Work out the finished part from the listing and answer in its coordinate system (mm). A direction names the side the tool comes from. Give positions to 0.01 mm unless a question says otherwise; leave off trailing zeros. Order: outer loops, then holes, each group sorted by start corner. A loop starts at its lowest first (then second) coordinate and runs counter-clockwise, first axis right, second up.
```python
from build123d import *

# Parameters (mm, degrees)
BOSS_EXTRUDE1_DEPTH = 1.2
FILLET1_R           = 4
FILLET2_R           = 2.5
BOSS_EXTRUDE2_DEPTH = 0.9
CUT_EXTRUDE1_DEPTH  = 0.9
CUT_EXTRUDE2_DEPTH  = 86.698804049


with BuildPart() as part:
    # Sketch1 → Boss-Extrude1 (new body)
    with BuildSketch(Plane(origin=(0, 0, 0), x_dir=(1, 0, 0), z_dir=(0, 1, 0))):
        Polygon((-59.653240417, 31.238807945), (-9.653240417, 31.238807945), (-9.653240417, 36.238807945), (-4.653240417, 36.238807945), (-4.653240417, 51.238807945), (-9.653240417, 51.238807945), (-9.653240417, 56.238807945), (-59.653240417, 56.238807945), (-59.653240417, 51.238807945), (-64.653240417, 51.238807945), (-64.653240417, 36.238807945), (-59.653240417, 36.238807945), align=None)
    extrude(amount=BOSS_EXTRUDE1_DEPTH)

    # Fillet1
    fillet1_edges = [part.edges().sort_by_distance(p)[0] for p in [
        (-59.653240417, 0.6, -56.238807945),
        (-9.653240417, 0.6, -56.238807945),
        (-9.653240417, 0.6, -31.238807945),
        (-59.653240417, 0.6, -31.238807945),
    ]]
    fillet(fillet1_edges, radius=FILLET1_R)

    # Fillet2
    fillet2_edges = [part.edges().sort_by_distance(p)[0] for p in [
        (-64.653240417, 0.6, -36.238807945),
        (-64.653240417, 0.6, -51.238807945),
        (-4.653240417, 0.6, -51.238807945),
        (-4.653240417, 0.6, -36.238807945),
    ]]
    fillet(fillet2_edges, radius=FILLET2_R)

    # Sketch4 → Boss-Extrude2 (add)
    with BuildSketch(Plane(origin=(0, 1.2, 0), x_dir=(1, 0, 0), z_dir=(0, 1, 0))):
        with BuildLine():
            Line((-59.153240417, 50.738807945), (-59.153240417, 36.738807945))
            Line((-59.153240417, 36.738807945), (-59.153240417, 35.238807945))
            ThreePointArc((-59.153240417, 35.238807945), (-58.128114151, 32.763934211), (-55.653240417, 31.738807945))
            Line((-55.653240417, 31.738807945), (-13.653240417, 31.738807945))
            ThreePointArc((-13.653240417, 31.738807945), (-11.178366683, 32.763934211), (-10.153240417, 35.238807945))
            Line((-10.153240417, 35.238807945), (-10.153240417, 36.738807945))
            Line((-10.153240417, 36.738807945), (-10.153240417, 50.738807945))
            Line((-10.153240417, 50.738807945), (-10.153240417, 52.238807945))
            ThreePointArc((-10.153240417, 52.238807945), (-11.178366683, 54.713681679), (-13.653240417, 55.738807945))
            Line((-13.653240417, 55.738807945), (-55.653240417, 55.738807945))
            ThreePointArc((-55.653240417, 55.738807945), (-58.128114151, 54.713681679), (-59.153240417, 52.238807945))
            Line((-59.153240417, 52.238807945), (-59.153240417, 50.738807945))
        make_face()
    extrude(amount=BOSS_EXTRUDE2_DEPTH)

    # Sketch5 → Cut-Extrude1 (cut)
    with BuildSketch(Plane(origin=(0, 2.1, 0), x_dir=(1, 0, 0), z_dir=(0, 1, 0))):
        with BuildLine():
            Line((-58.553240417, 52.238807945), (-58.553240417, 35.238807945))
            ThreePointArc((-58.553240417, 35.238807945), (-57.703850082, 33.18819828), (-55.653240417, 32.338807945))
            Line((-55.653240417, 32.338807945), (-13.653240417, 32.338807945))
            ThreePointArc((-13.653240417, 32.338807945), (-11.602630751, 33.18819828), (-10.753240417, 35.238807945))
            Line((-10.753240417, 35.238807945), (-10.753240417, 52.238807945))
            ThreePointArc((-10.753240417, 52.238807945), (-11.602630751, 54.289417611), (-13.653240417, 55.138807945))
            Line((-13.653240417, 55.138807945), (-55.653240417, 55.138807945))
            ThreePointArc((-55.653240417, 55.138807945), (-57.703850082, 54.289417611), (-58.553240417, 52.238807945))
        make_face()
    extrude(amount=-CUT_EXTRUDE1_DEPTH, mode=Mode.SUBTRACT)

    # Sketch6 → Cut-Extrude2 (cut, through all)
    with BuildSketch(Plane(origin=(0, 1.2, 0), x_dir=(1, 0, 0), z_dir=(0, 1, 0))):
        with BuildLine():
            Line((-63.153240417, 48.738807945), (-63.153240417, 38.738807945))
            ThreePointArc((-63.153240417, 38.738807945), (-62.153240417, 37.738807945), (-61.153240417, 38.738807945))
            Line((-61.153240417, 38.738807945), (-61.153240417, 48.738807945))
            ThreePointArc((-61.153240417, 48.738807945), (-62.153240417, 49.738807945), (-63.153240417, 48.738807945))
        make_face()
        with BuildLine():
            Line((-8.153185775, 48.728354232), (-8.153240417, 38.738807945))
            ThreePointArc((-8.153240417, 38.738807945), (-7.153245887, 37.738807945), (-6.153240417, 38.738807945))
            Line((-6.153240417, 38.738807945), (-6.153240417, 48.738807945))
            ThreePointArc((-6.153240417, 48.738807945), (-7.158467345, 49.738794285), (-8.153185775, 48.728354232))
        make_face()
    extrude(amount=-CUT_EXTRUDE2_DEPTH, mode=Mode.SUBTRACT)


solid = part.part
```
1. The part is cut by section C-C (z = -54.25). Write down the section's boundary in (x, y), then the cut area to 3 significant figures.
Findings below:
outline: (-59.11, 0) - (-10.2, 0) - (-10.2, 1.2) - (-10.79, 1.2) - (-10.79, 2.1) - (-11.56, 2.1) - (-11.56, 1.2) - (-57.74, 1.2) - (-57.74, 2.1) - (-58.52, 2.1) - (-58.52, 1.2) - (-59.11, 1.2) - close
area: 60.1 mm2
2. The part is cut by section A-A (y = 0.4). Write down the section's boundary in (x, z).
Findings below:
outline: (-64.65, -48.74) arc R2.5 ccw to (-62.15, -51.24) - (-59.65, -51.24) - (-59.65, -52.24) arc R4 ccw to (-55.65, -56.24) - (-13.65, -56.24) arc R4 ccw to (-9.65, -52.24) - (-9.65, -51.24) - (-7.15, -51.24) arc R2.5 ccw to (-4.65, -48.74) - (-4.65, -38.74) arc R2.5 ccw to (-7.15, -36.24) - (-9.65, -36.24) - (-9.65, -35.24) arc R4 ccw to (-13.65, -31.24) - (-55.65, -31.24) arc R4 ccw to (-59.65, -35.24) - (-59.65, -36.24) - (-62.15, -36.24) arc R2.5 ccw to (-64.65, -38.74) - close; hole (-63.15, -48.74) arc R1 ccw to (-61.15, -48.74) - (-61.15, -38.74) arc R1 ccw to (-63.15, -38.74) - close; hole (-8.15, -48.73) arc R1 ccw (long way) to (-6.15, -48.74) - (-6.15, -38.74) arc R1 ccw to (-8.15, -38.74) - close
3. The part is cut by section D-D (z = -45.25). Write down the section's boundary in (x, y).
Findings below:
outline: (-64.65, 0) - (-63.15, 0) - (-63.15, 1.2) - (-64.65, 1.2) - close; (-61.15, 0) - (-8.15, 0) - (-8.15, 1.2) - (-10.15, 1.2) - (-10.15, 2.1) - (-10.75, 2.1) - (-10.75, 1.2) - (-58.55, 1.2) - (-58.55, 2.1) - (-59.15, 2.1) - (-59.15, 1.2) - (-61.15, 1.2) - close; (-6.15, 0) - (-4.65, 0) - (-4.65, 1.2) - (-6.15, 1.2) - close
4. The mould has two halves that part along Z. Classify faces 6 (the face through (-10.794, 0.608, -55.036)), 7 (the face through (-62.13, 0.61, -49.74)), 8 (the face through (-8, 1, -36.239)): pulls with the +Z half, pulls with the -Z half, needs draft (parallel to the pull), parting line crosses it, or undercut.
Findings below:
face 6: pulls with the -Z half
face 7: undercut
face 8: pulls with the +Z half
5. The part is cut by section B-B (x = -28). Write down the section's boundary in (y, z), then the cut area to 3 significant figures.
Findings below:
outline: (0, -56.24) - (1.2, -56.24) - (1.2, -55.74) - (2.1, -55.74) - (2.1, -55.14) - (1.2, -55.14) - (1.2, -32.34) - (2.1, -32.34) - (2.1, -31.74) - (1.2, -31.74) - (1.2, -31.24) - (0, -31.24) - close
area: 31.1 mm2
6. Given P1, Ø0.6, axis at x = -61, y = 1, coming from the -Z side; P2, Ø0.5, axis at x = -34.5, y = 1.5, coming from the +Z side; P3, Ø1, axis at x = -26, z = -45, coming from the +Y side, each flat-ended and moving along its own axis, determine where each tip first touches the part or whether it passes through.
Findings below:
P1: stops at z = -51.24
P2: stops at z = -31.74
P3: stops at y = 1.2
7. Which of the six approach directions +Z, -Z, +X, -X, +Y, -Y give full straight-line access (tool end or side, diameter ignored) to faces 1 (the face through (-7.18, 0.61, -37.74)), 2 (the face through (-11.206, 1.644, -32.737)), 3 (the face through (-61, 1, -51.239)), 4 (the face through (-11.151, 1.644, -54.686)), 5 (the face through (-35, 1.2, -44))?
Findings below:
face 1: +Y, -Y
face 2: +Z, +X, +Y
face 3: -Z, -X, +Y, -Y
face 4: -Z, +X, +Y
face 5: +Y
8. Straight lines are drawn through the part: probe 1 along X at (y, z) = (0.1, -40.75); probe 2 along Z at (x, y) = (-28, 1.6); probe 3 along X at (y, z) = (1.9, -50.75). For each, find the intervals that lie inside material, in ascending order.
Findings below:
probe 1: x = -64.65 to -63.15, -61.15 to -8.15, -6.15 to -4.65
probe 2: z = -55.74 to -55.14, -32.34 to -31.74
probe 3: x = -59.15 to -58.55, -10.75 to -10.15
